Part model, mm, in its own coordinate system. Give positions to 0.01 mm unless a question says otherwise; leave off trailing zeros. Order: outer loops, then holes, each group sorted by start corner. A loop starts at its lowest first (then second) coordinate and runs counter-clockwise, first axis right, second up.
1. Slice it at B-B on y = -9.25. List the corners of the cut face in (x, z), and give its area (3 significant figures).
2. Drop a flat-ended pin along its axis: pin 1 Ø2 at (y, z) = (9, 4.5) entering from -X. Give the stop position or say it passes through.
3. Probe line 1 (Y direction, x = 8, z = 3.85); line 2 (X direction, y = -9.75, z = 4.3); line 3 (Y direction, x = -0.5, z = 3.25). List the from-to ranges inside material, lowest first.
4. Slice it at D-D on x = 5.5. List the corners of the cut face in (y, z), and give its area (3 significant figures).
5. Slice it at C-C on x = -11. List the corners of the cut face in (y, z).
6. Slice it at A-A on x = 0. List the corners of the cut face in (y, z), and give its area (3 significant figures).
from build123d import *

# Parameters (mm, degrees)
SKETCH1_R           = 13.2
SKETCH1_R_2         = 6
BOSS_EXTRUDE1_DEPTH = 6
CUT_EXTRUDE1_DEPTH  = 7
CIRPATTERN2_COUNT   = 14


with BuildPart() as part:
    # Sketch1 → Boss-Extrude1 (new body)
    with BuildSketch(Plane.XY):
        Circle(SKETCH1_R)
        Circle(SKETCH1_R_2, mode=Mode.SUBTRACT)
    extrude(amount=BOSS_EXTRUDE1_DEPTH)

    # Sketch2 → Cut-Extrude1 (cut, through all)
    with BuildSketch(Plane.XY.offset(6)):
        with BuildLine():
            ThreePointArc((-2.819851171, 12.895287487), (0, 13.2), (2.819851171, 12.895287487))
            ThreePointArc((2.819851171, 12.895287487), (1.826256171, 11.910750525), (1.819851171, 10.512))
            ThreePointArc((1.819851171, 10.512), (0, 10.668364555), (-1.819851171, 10.512))
            ThreePointArc((-1.819851171, 10.512), (-1.826256171, 11.910750525), (-2.819851171, 12.895287487))
        make_face()
    cut_extrude1 = extrude(amount=-CUT_EXTRUDE1_DEPTH, mode=Mode.SUBTRACT)

    # CirPattern2: Cut-Extrude1 ×14 about axis
    cirpattern2_axis = Axis((0, 0, 0), (0, 0, 1))
    for i in range(1, CIRPATTERN2_COUNT):
        add(cut_extrude1.rotate(cirpattern2_axis, i * 360 / CIRPATTERN2_COUNT), mode=Mode.SUBTRACT)


solid = part.part
Data:
1. outline: (-8.33, 0) - (-6.33, 0) - (-6.33, 6) - (-8.33, 6) - close; (-5.32, 0) - (5.32, 0) - (5.32, 6) - (-5.32, 6) - close; (6.33, 0) - (8.33, 0) - (8.33, 6) - (6.33, 6) - close
1. area: 87.8 mm2
2. pin 1: stops at x = -8.4
3. line 1: y = -10.4 to -8.59, -7.06 to 7.06, 8.59 to 10.4
3. line 2: x = -8.4 to -6.63, -4.33 to 4.33, 6.63 to 8.4
3. line 3: y = -10.66 to -5.98, 5.98 to 10.66
4. outline: (-9.14, 0) - (-2.4, 0) - (-2.4, 6) - (-9.14, 6) - close; (2.4, 0) - (9.14, 0) - (9.14, 6) - (2.4, 6) - close
4. area: 80.9 mm2
5. outline: (-6.07, 0) - (-4.3, 0) - (-4.3, 6) - (-6.07, 6) - close; (-0.76, 0) - (0.76, 0) - (0.76, 6) - (-0.76, 6) - close; (4.3, 0) - (6.07, 0) - (6.07, 6) - (4.3, 6) - close
6. outline: (-10.67, 0) - (-6, 0) - (-6, 6) - (-10.67, 6) - close; (6, 0) - (10.67, 0) - (10.67, 6) - (6, 6) - close
6. area: 56.0 mm2
